Could you check a few things on this model? Use its own coordinates, in mm. Round coordinates to 2 decimals unless told otherwise and drop trailing zeros. Loops run counter-clockwise (first coordinate to the right, second up) from the corner with the lowest first, then second, coordinate; pieces in that order, holes last. Notation, with made-up numbers: (88, -23) -> (145, -23) arc R24 cw to (145, -4) -> close; hole circle Ø10 at (-38.75, -25). An arc over 180 degrees is marked (long way). Write each question's results on one line, items separated by ' | '. Start each with the question number.
1) Imagine slicing it at A-A, the plane x = 0. List the corners of the cut face in (y, z) for me.
2) For P1, Ø2, axis at y = 1.5, z = 1, coming from the +X side; P2, Ø4.5, axis at x = 0, y = 17, coming from the -Z side, each with a flat end and sliding along its axis, tell me the tip position at first contact or that it passes through.
3) Imagine slicing it at B-B, the plane z = 2.25. List the corners of the cut face in (x, y) for me, plus the area to 3 significant figures.
4) We'd pull the mould along X, two halves only. Please class faces 1 (the flat face through (0, 11, 4)), 2 (the cylindrical face through (1.246, 6.395, 1.726)), 3 (the cylindrical face through (0, -2, 2)): pulls with the +X half, pulls with the -X half, needs draft (parallel to the pull), parting line crosses it, or undercut.
5) If I drill on probe 1 along Y at (x, z) = (0, 1.8); probe 2 along X at (y, z) = (17.5, 3.1); probe 3 along X at (y, z) = (4.75, 3.65), over which ranges is the centre line in solid material (lowest first)?
Solid Edge part; units mm, degrees
sketch "Sketch1" plane through (0, 0, 0) normal (0, 0, 1) x (1, 0, 0)
  circle A0 centre (0, 4) radius 2.7
  line L0 (-6, 17) -> (-6, 4)
  line L1 (6, 17) -> (6, 4)
  arc A1 (6, 17) -> (-6, 17) centre (0, 17) ccw
  arc A2 (-6, 4) -> (6, 4) centre (0, 4) ccw
  circle A3 centre (0, 17) radius 2.7
extrude "Protrusion1" add sketch "Sketch1" along normal blind 4
chamfer "Chamfer_1" [suppressed]
chamfer "Chamfer_2" distance 0.5 angle 45 6 edges at (0, -2, 4) (6, 10.5, 4) (0, 23, 4) (-6, 10.5, 4) (-2.7, 4, 4) (-2.7, 17, 4)
properties material "ABS Plastic, medium impact"
Checked values:
1) outline: (-2, 0) -> (1.3, 0) -> (1.3, 3.5) -> (0.8, 4) -> (-1.5, 4) -> (-2, 3.5) -> close; (6.7, 0) -> (14.3, 0) -> (14.3, 3.5) -> (13.8, 4) -> (7.2, 4) -> (6.7, 3.5) -> close; (19.7, 0) -> (23, 0) -> (23, 3.5) -> (22.5, 4) -> (20.2, 4) -> (19.7, 3.5) -> close
2) P1: x = 5.81 | P2: through
3) outline: (-6, 4) arc R6 ccw to (6, 4) -> (6, 17) arc R6 ccw to (-6, 17) -> close; hole circle Ø5.4 at (0, 4); hole circle Ø5.4 at (0, 17) | area: 223 mm^2
4) face 1: needs draft | face 2: undercut | face 3: parting line crosses it
5) probe 1: -2 to 1.3, 6.7 to 14.3, 19.7 to 23 | probe 2: -5.98 to -2.65, 2.65 to 5.98 | probe 3: -5.85 to -2.75, 2.75 to 5.85
